Autodesk Inventor part; units mm, degrees
ref_plane "YZ Plane" through (0, 0, 0) normal (1, 0, 0) x (0, 1, 0)
ref_plane "XZ Plane" through (0, 0, 0) normal (0, 1, 0) x (-1, 0, 0)
ref_plane "XY Plane" through (0, 0, 0) normal (0, 0, 1) x (1, 0, 0)
sketch "Эскиз1" plane through (0, 0, 0) normal (0, 1, 0) x (-1, 0, 0)
  line L0 (90, -180) -> (-90, -180)
  line L1 (-90, -180) -> (-90, 180)
  line L2 (-90, 180) -> (90, 180)
  line L3 (90, 180) -> (90, -180)
  line L4 (90, -180) -> (-90, 180) construction
  line L5 (-90, -180) -> (90, 180) construction
  point P0 (0, 0)
  dimension "d0" = 180
  dimension "d1" = 360
extrude "Выдавливание1" add sketch "Эскиз1" along normal blind 10
fillet "Сопряжение1" radius 10 4 edges at (-90, 5, -180) (-90, 5, 180) (90, 5, 180) (90, 5, -180)
sketch "Эскиз2" plane through (0, 10, 0) normal (0, 1, 0) x (1, 0, 0)
  line L0 (90, -170) -> (90, 170)
  line L1 (-80, -180) -> (80, -180)
  line L2 (0, 185.9906) -> (0, -228.4226) construction
  line L3 (-161.892, 0) -> (248.2378, 0) construction
  point P0 (0, 0)
  point P1 (75, -165)
  point P2 (75, 0)
  point P3 (0, -165)
  point P4 (75, 165)
  point P5 (0, 165)
  point P6 (-75, -165)
  point P7 (-75, 0)
  point P8 (-75, 165)
  point P9 (90, 0)
  dimension "d5" = 15
  dimension "d7" = 15
hole "Отверстие1" at (75, 10, 165) at (75, 10, 0) at (0, 10, 165) at (0, 10, -165) at (75, 10, -165) at (-75, 10, -165) at (-75, 10, 0) at (-75, 10, 165) direction (0, -1, 0) diameter 8.376 end through all
sketch "Эскиз3" plane through (0, 10, 0) normal (0, 1, 0) x (1, 0, 0)
  circle A0 centre (0, 0) radius 20
  dimension "d15" = 40
extrude "Выдавливание2" cut sketch "Эскиз3" against normal through all
properties part number "МПСТ люк" material "Сталь, углеродистая"
Here's how the part is built. I have some questions about the finished solid (model axes, mm). Round coordinates to 2 decimals unless told otherwise and drop trailing zeros. Order: outer loops, then holes, each group sorted by start corner. A loop starts at its lowest first (then second) coordinate and runs counter-clockwise, first axis right, second up. Notation, with made-up numbers: M 56.25,-16.75 L 107.25,-16.75 A25 cw 107.25,3.25 Z; hole C 12,30.5 d10. An arc over 180 degrees is marked long. Return JSON: item names as keys, results as strings. Group by question number.
1. If we section it at C-C on z = 165: List the corners of the cut face in (x, y) for me.
2. If we mould it in two halves opening along X, with no side actions, what happens to faces 1 (the face through (-1, 5, -180)), 2 (the face through (-75.184, 4.93, 160.816)), 3 (the face through (-87.15, 5.07, 176.99))? For each: pulls with the +X half, pulls with the -X half, needs draft (parallel to the pull), parting line crosses it, or undercut.
3. Please list where these lines run through material, in increasing order: probe 1 along X at (y, z) = (6.5, 165); probe 2 along Z at (x, y) = (75, 6); probe 3 along X at (y, z) = (7, 1).
4. If we section it at B-B on x = 75: List the corners of the cut face in (y, z) for me.
5. If we section it at A-A on y = 8.5: State how many separate pieces and enclosed holes the cut face has, then the cut area to 3 significant figures.
Reply:
{
 "1": {"outline": "M -90,0 L -79.19,0 L -79.19,10 L -90,10 Z; M -70.81,0 L -4.19,0 L -4.19,10 L -70.81,10 Z; M 4.19,0 L 70.81,0 L 70.81,10 L 4.19,10 Z; M 79.19,0 L 90,0 L 90,10 L 79.19,10 Z"},
 "2": {"face 1": "needs draft", "face 2": "undercut", "face 3": "pulls with the -X half"},
 "3": {"probe 1": "-90 to -79.19, -70.81 to -4.19, 4.19 to 70.81, 79.19 to 90", "probe 2": "-180 to -169.19, -160.81 to -4.19, 4.19 to 160.81, 169.19 to 180", "probe 3": "-90 to -79.07, -70.93 to -19.97, 19.97 to 70.93, 79.07 to 90"},
 "4": {"outline": "M 0,-180 L 10,-180 L 10,-169.19 L 0,-169.19 Z; M 0,-160.81 L 10,-160.81 L 10,-4.19 L 0,-4.19 Z; M 0,4.19 L 10,4.19 L 10,160.81 L 0,160.81 Z; M 0,169.19 L 10,169.19 L 10,180 L 0,180 Z"},
 "5": {"separate pieces": "1", "enclosed holes": "9", "area": "63,000 mm^2"}
}
